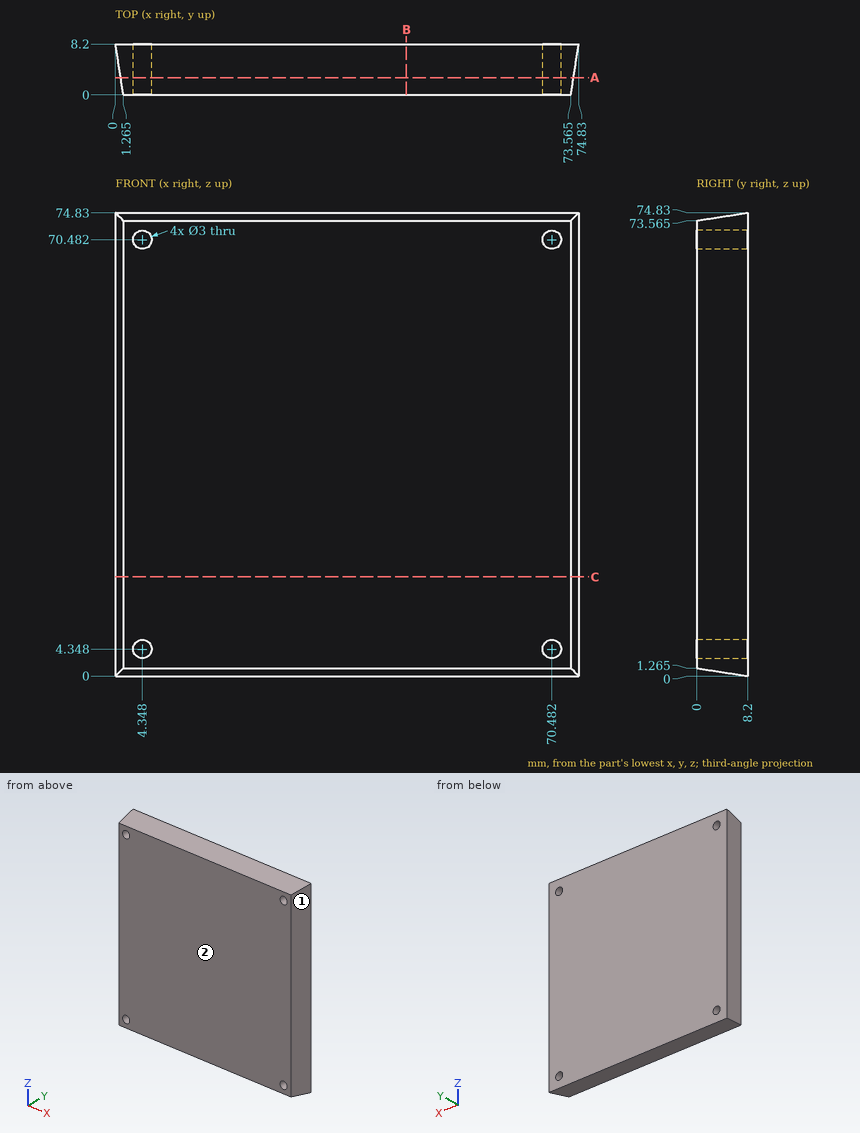
Here's the drawing with two shaded views (mm, measured from the low corner). I have some questions. Give positions to 0.01 mm unless a question says otherwise; leave off trailing zeros. Order: outer loops, then holes, each group sorted by start corner. A loop starts at its lowest first (then second) coordinate and runs counter-clockwise, first axis right, second up. Notation, with made-up numbers: M -20.75,-16 L 28.25,-16 A7 cw 28.25,-11 Z; hole C 6.25,4 d1. An arc over 180 degrees is marked long. Answer as a JSON object with one key per item and string values. Group by question number.
1) Suppose I cut it at C-C, the plane z = 16. Write out the boundary of the cut face in (x, y) (1 decimal), plus the area to 3 significant figures.
2) Please list where these lines run through material, in increasing order: L1, parallel to X at y = 0.75, z = 5; L2, parallel to X at y = 1, z = 51; L3, parallel to Z at x = 44, y = 7.25. Write a range as [from, to].
3) We'd pull the mould along X, two halves only. Please class the marked faces 1 and 2: pulls with the +X half, pulls with the -X half, needs draft (parallel to the pull), parting line crosses it, or undercut.
4) Suppose I cut it at B-B, the plane x = 47. Write out the boundary of the cut face in (y, z) (1 decimal).
5) I'm going to push flat-ended pins straight in: pin 1 Ø1.8 at (x, z) = (70.48, 70.48) entering from +Y; pin 2 Ø3 at (x, y) = (58, 5) entering from +Z; pin 3 Ø4 at (x, y) = (52.5, 2.5) entering from +Z; pin 4 Ø1.5 at (x, y) = (58.5, 5) entering from +Z. Where does each tip first touch, or does it pass through?
6) Suppose I cut it at A-A, the plane y = 2.75. Write out the boundary of the cut face in (x, z), plus the area to 3 significant figures.
Results found:
{
 "1": {"outline": "M 0,8.2 L 1.3,0 L 73.6,0 L 74.8,8.2 Z", "area": "603 mm²"},
 "2": {"L1": "[1.15, 3], [5.7, 69.13], [71.83, 73.68]", "L2": "[1.11, 73.72]", "L3": "[0.15, 74.68]"},
 "3": {"face 1": "pulls with the +X half", "face 2": "needs draft"},
 "4": {"outline": "M 0,1.3 L 8.2,0 L 8.2,74.8 L 0,73.6 Z"},
 "5": {"pin 1": "through", "pin 2": "z = 74.57", "pin 3": "z = 74.26", "pin 4": "z = 74.45"},
 "6": {"outline": "M 0.84,0.84 L 73.99,0.84 L 73.99,73.99 L 0.84,73.99 Z; hole C 4.35,4.35 d3; hole C 4.35,70.48 d3; hole C 70.48,4.35 d3; hole C 70.48,70.48 d3", "area": "5,320 mm²"}
}
